The listing builds one solid part. Answer for the finished solid, in the listing's coordinates (mm). Face numbers are marked on the shaded views. A direction names the side the tool comes from. Round coordinates to 2 decimals unless told otherwise and drop trailing zeros. Write each loop counter-clockwise with the first axis right and the second up, starting at its lowest first coordinate (ties: lowest second). Pieces come first, ordered by that corner, then holes. Notation, with made-up numbers: M -17.5,50 L 19.5,50 A15 cw 19.5,58 Z; hole C 7,-1 d1. An arc over 180 degrees is marked long. One line per item, written item: value. Start each with the question number.
(1) Consider probe 1 along Z at (x, y) = (-8.5, 11.1) (3 decimals); probe 2 along Z at (x, y) = (-2.5, 78) (3 decimals); probe 3 along Y at (x, z) = (-2.5, -27.5). Determine where each line is inside the solid, lowest interval first.
(2) For a pull along Y with two mould halves and no side action, classify the marked faces 1, 2 and 3 as released by +Y, released by -Y, zero draft, split by the parting line, or undercut.
(3) Section B-B (y = 59.5) is taken. Determine the outline of the cut face in (x, z) (3 decimals).
(4) Given P1, Ø8, axis at x = 1.5, z = 14, coming from the -Y side; P2, Ø5, axis at x = 1, z = -28.5, coming from the -Y side; P3, Ø5.5, axis at x = -9.5, y = 13, coming from the -Z side; P4, Ø0.9, axis at x = -0.5, y = 5.5, coming from the +Z side, each flat-ended and moving along its own axis, determine where each tip first touches the part or whether it passes through.
(5) For the marked faces 4, 5 and 6, determine the directions among +Z, -Z, +X, -X, +Y, -Y from which every point of the face is accessible in a straight line to the end or side of a thin tool.
(6) Section D-D (x = 0) is taken. Determine the outline of the cut face in (y, z) (3 decimals), plus the area to 3 significant figures.
(7) Section A-A (z = -11.5) is taken. Determine the outline of the cut face in (x, y).
(8) Section C-C (x = -8.5) is taken. Determine the outline of the cut face in (y, z) (3 decimals), plus the area to 3 significant figures.
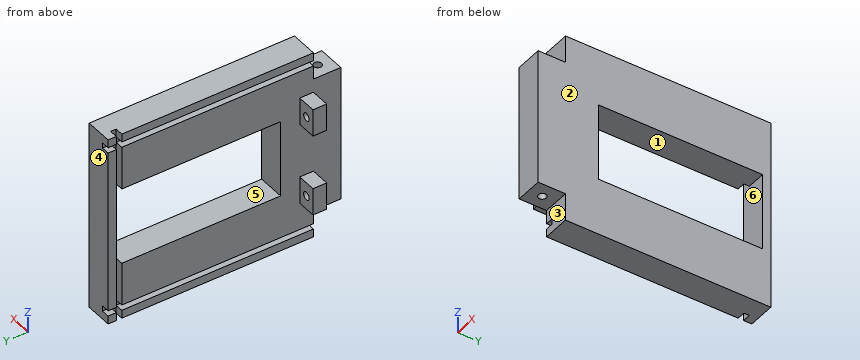
```python
from build123d import *

# Parameters (mm, degrees)
CROQUIS1_W              = 10
CROQUIS1_H              = 70
SALIENTE_EXTRUIR1_DEPTH = 10
CROQUIS8_W              = 10
CROQUIS8_H              = 70
SALIENTE_EXTRUIR3_DEPTH = 75
CROQUIS9_W              = 2
CROQUIS9_H              = 75
CORTAR_EXTRUIR4_DEPTH   = 3
CROQUIS10_W             = 70
CROQUIS10_H             = 2
CORTAR_EXTRUIR5_DEPTH   = 3
CORTAR_EXTRUIR6_REACH   = 12
CROQUIS11_W             = 28.25
CROQUIS11_H             = 60
CROQUIS16_W             = 10
CROQUIS16_H             = 5
SALIENTE_EXTRUIR5_DEPTH = 7
CROQUIS17_R             = 1.435
CORTAR_EXTRUIR9_DEPTH   = 5
CROQUIS18_W             = 10
CROQUIS18_H             = 10
CORTAR_EXTRUIR10_DEPTH  = 10
CROQUIS19_R             = 1.435
CORTAR_EXTRUIR11_DEPTH  = 10


with BuildPart() as part:
    # Croquis1 → Saliente-Extruir1 (new body)
    with BuildSketch(Plane(origin=(0, 0, 0), x_dir=(1, 0, 0), z_dir=(0, 1, 0))):
        Rectangle(CROQUIS1_W, CROQUIS1_H)
    extrude(amount=SALIENTE_EXTRUIR1_DEPTH)

    # Croquis8 → Saliente-Extruir3 (add)
    with BuildSketch(Plane(origin=(0, 10, 0), x_dir=(1, 0, 0), z_dir=(0, 1, 0))):
        Rectangle(CROQUIS8_W, CROQUIS8_H)
    extrude(amount=SALIENTE_EXTRUIR3_DEPTH)

    # Croquis9 → Cortar-Extruir4 (cut)
    with BuildSketch(Plane.ZY.offset(5)):
        with Locations((-31, 47.5)):
            Rectangle(CROQUIS9_W, CROQUIS9_H)
    cortar_extruir4 = extrude(amount=-CORTAR_EXTRUIR4_DEPTH, mode=Mode.SUBTRACT)

    # Simetría2: Cortar-Extruir4 across plane
    add(cortar_extruir4.mirror(Plane.XY), mode=Mode.SUBTRACT)

    # Croquis10 → Cortar-Extruir5 (cut)
    with BuildSketch(Plane.ZY.offset(5)):
        with Locations((0, 81)):
            Rectangle(CROQUIS10_W, CROQUIS10_H)
    extrude(amount=-CORTAR_EXTRUIR5_DEPTH, mode=Mode.SUBTRACT)

    # Croquis11 → Cortar-Extruir6 (cut, up to next)
    with BuildSketch(Plane.ZY.offset(5), mode=Mode.PRIVATE) as cortar_extruir6_sk1:
        with Locations((0, 52)):
            Rectangle(CROQUIS11_W, CROQUIS11_H)
    cortar_extruir6_tool1 = extrude(cortar_extruir6_sk1.sketch, amount=-CORTAR_EXTRUIR6_REACH, mode=Mode.PRIVATE) & part.part
    add(cortar_extruir6_tool1.solids().sort_by_distance((-5, 52, 0))[0], mode=Mode.SUBTRACT)

    # Croquis16 → Saliente-Extruir5 (add)
    with BuildSketch(Plane.ZY.offset(5)):
        with Locations((-15, 12.5)):
            Rectangle(CROQUIS16_W, CROQUIS16_H)
    saliente_extruir5 = extrude(amount=SALIENTE_EXTRUIR5_DEPTH)

    # Simetría5: Saliente-Extruir5 across plane
    add(saliente_extruir5.mirror(Plane.XY))

    # Croquis17 → Cortar-Extruir9 (cut)
    with BuildSketch(Plane(origin=(0, 15, 0), x_dir=(1, 0, 0), z_dir=(0, 1, 0))):
        with Locations((-8.5, 15)):
            Circle(CROQUIS17_R)
    cortar_extruir9 = extrude(amount=-CORTAR_EXTRUIR9_DEPTH, mode=Mode.SUBTRACT)

    # Simetría6: Cortar-Extruir9 across plane
    add(cortar_extruir9.mirror(Plane.XY), mode=Mode.SUBTRACT)

    # Croquis18 → Cortar-Extruir10 (cut)
    with BuildSketch(Plane.ZY.offset(5)):
        with Locations((-30, 5)):
            Rectangle(CROQUIS18_W, CROQUIS18_H)
    cortar_extruir10 = extrude(amount=-CORTAR_EXTRUIR10_DEPTH, mode=Mode.SUBTRACT)

    # Simetría7: Cortar-Extruir10 across plane
    add(cortar_extruir10.mirror(Plane.XY), mode=Mode.SUBTRACT)

    # Croquis19 → Cortar-Extruir11 (cut)
    with BuildSketch(Plane(origin=(0, 0, -25), x_dir=(-1, 0, 0), z_dir=(0, 0, -1))):
        with Locations((0, 5)):
            Circle(CROQUIS19_R)
    cortar_extruir11 = extrude(amount=-CORTAR_EXTRUIR11_DEPTH, mode=Mode.SUBTRACT)

    # Simetría8: Cortar-Extruir11 across plane
    add(cortar_extruir11.mirror(Plane.XY), mode=Mode.SUBTRACT)


solid = part.part
```
Recorded:
1. probe 1: z = -20 to -16.435, -13.565 to -10, 10 to 13.565, 16.435 to 20
1. probe 2: z = -35 to -32, -30 to -14.125, 14.125 to 30, 32 to 35
1. probe 3: y = 10 to 80, 82 to 85
2. face 1: undercut
2. face 2: zero draft
2. face 3: released by -Y
3. outline: M -5,-35 L 5,-35 L 5,-14.125 L -5,-14.125 L -5,-30 L -2,-30 L -2,-32 L -5,-32 Z; M -5,14.125 L 5,14.125 L 5,35 L -5,35 L -5,32 L -2,32 L -2,30 L -5,30 Z
4. P1: stops at y = 0
4. P2: stops at y = 10
4. P3: stops at z = -20
4. P4: stops at z = 15
5. face 4: +Z, -Z, +X, -X, +Y
5. face 5: +X, -X
5. face 6: -X
6. outline: M 0,-25 L 3.565,-25 L 3.565,-15 L 6.435,-15 L 6.435,-25 L 10,-25 L 10,-35 L 85,-35 L 85,35 L 10,35 L 10,25 L 6.435,25 L 6.435,15 L 3.565,15 L 3.565,25 L 0,25 Z; hole M 22,-14.125 L 82,-14.125 L 82,14.125 L 22,14.125 Z
6. area: 4,000 mm2
7. outline: M -12,10 L -5,10 L -5,0 L 5,0 L 5,22 L -5,22 L -5,15 L -12,15 Z; M -5,82 L 5,82 L 5,85 L -5,85 Z
8. outline: M 10,-20 L 15,-20 L 15,-16.435 L 10,-16.435 Z; M 10,-13.565 L 15,-13.565 L 15,-10 L 10,-10 Z; M 10,10 L 15,10 L 15,13.565 L 10,13.565 Z; M 10,16.435 L 15,16.435 L 15,20 L 10,20 Z
8. area: 71.3 mm2
